Input: part model. Units: mm. Frame: model coordinates. Coordinates: 2 decimals unless noted, no trailing zeros. Write each loop counter-clockwise with the first axis right and the second up, starting at its lowest first coordinate (ties: lowest second). Pieces come first, ordered by that corner, then holes. Notation, with made-up numbers: (59.5, 5) - (74.5, 5) arc R24 cw to (74.5, 35) - close; hole circle Ø7 at (16.25, 21). An arc over 180 degrees is marked (long way). Use CSV: the item, a comma, the result in double quotes.
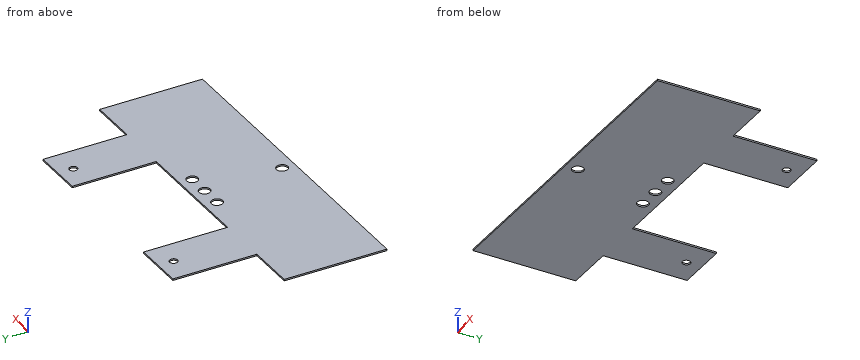
```python
from build123d import *

# Parameters (mm, degrees)
BOSS_EXTRUDE1_DEPTH = 0.6096
SKETCH5_R           = 2.25
CUT_EXTRUDE2_DEPTH  = 430.420105
SKETCH6_R           = 1.5875
CUT_EXTRUDE5_DEPTH  = 0.6096
SKETCH7_R           = 1.5875
CUT_EXTRUDE6_DEPTH  = 0.6096
SKETCH8_R           = 2.25
CUT_EXTRUDE7_DEPTH  = 2.54


with BuildPart() as part:
    # Sketch1 → Boss-Extrude1 (new body)
    with BuildSketch(Plane(origin=(16.997226787, -4.149929847, 204.631375634), x_dir=(0.99656941, 0.00195951, -0.082737969), z_dir=(-0.082760694, 0.020206301, -0.996364578))):
        Polygon((-405.631572024, 283.216979703), (-385.692572024, 283.216979703), (-385.692572024, 323.856979703), (-405.014358213, 323.856979703), (-432.414358217, 323.856979703), (-445.097076418, 323.856979703), (-465.359895626, 323.856979703), (-479.498480719, 323.856979703), (-500.373572024, 323.856979703), (-520.312572024, 323.856979703), (-520.312572024, 283.216979703), (-500.373572024, 283.216979703), (-500.373572024, 250.003685703), (-479.037572024, 250.003685703), (-479.037572024, 283.216979703), (-426.967572024, 283.216979703), (-426.967572024, 250.003685703), (-405.631572024, 250.003685703), align=None)
    extrude(amount=BOSS_EXTRUDE1_DEPTH)

    # Sketch5 → Cut-Extrude2 (cut)
    with BuildSketch(Plane(origin=(16.946775868, -4.137612086, 204.023991787), x_dir=(-0.996569449, -0.001678044, 0.082743681), z_dir=(-0.082760694, 0.020206301, -0.996364578))):
        with Locations((452.956635294, -318.984510283)):
            Circle(SKETCH5_R)
    cut_extrude2 = extrude(amount=-CUT_EXTRUDE2_DEPTH, mode=Mode.SUBTRACT)

    # Mirror1: Cut-Extrude2 across plane
    add(cut_extrude2.mirror(Plane(origin=(0.085159645, -303.474424262, -6.16154314), x_dir=(5.696e-06, -0.020299151, 0.999793951), z_dir=(0.000280558, -0.999793912, -0.020299152))), mode=Mode.SUBTRACT)

    # Sketch6 → Cut-Extrude5 (cut)
    with BuildSketch(Plane(origin=(16.946775868, -4.137612086, 204.023991787), x_dir=(-0.996569449, -0.001678044, 0.082743681), z_dir=(-0.082760694, 0.020206301, -0.996364578))):
        with Locations((416.50680125, -256.173836565)):
            Circle(SKETCH6_R)
    extrude(amount=-CUT_EXTRUDE5_DEPTH, mode=Mode.SUBTRACT)

    # Sketch7 → Cut-Extrude6 (cut)
    with BuildSketch(Plane(origin=(16.946775868, -4.137612086, 204.023991787), x_dir=(-0.996569449, -0.001678044, 0.082743681), z_dir=(-0.082760694, 0.020206301, -0.996364578))):
        with Locations((489.681466673, -256.194436956)):
            Circle(SKETCH7_R)
    extrude(amount=-CUT_EXTRUDE6_DEPTH, mode=Mode.SUBTRACT)

    # Sketch8 → Cut-Extrude7 (cut)
    with BuildSketch(Plane(origin=(16.997226787, -4.149929847, 204.631375634), x_dir=(0.996569449, 0.001678044, -0.082743681), z_dir=(0.082760694, -0.020206301, 0.996364578))):
        with Locations((-443.925718519, -288.341966658)):
            Circle(SKETCH8_R)
        with Locations((-960.270444462, 120.825542597)):
            Circle(SKETCH8_R)
        with Locations((-462.00480383, -288.347056346)):
            Circle(SKETCH8_R)
    extrude(amount=-CUT_EXTRUDE7_DEPTH, mode=Mode.SUBTRACT)


solid = part.part
```
(1) Cut plane B-B on x = -476. Return loops of the section in (y, z).
Check values:
outline,"(-328.91, 238.99) - (-328.9, 238.38) - (-255.06, 239.88) - (-255.07, 240.49) - close"
(2) Cut plane C-C on y = -312. Return loops of the section in (x, z), and give its area (3 significant figures).
Check values:
outline,"(-501.49, 240.84) - (-367.34, 229.7) - (-367.29, 230.31) - (-501.44, 241.45) - close"
area,"82.1 mm^2"
(3) Pin query (flat end, axial travel): pin 1 Ø1 at (x, z) = (-437.5, 236) entering from +Y; pin 2 Ø6 at (y, z) = (-264.5, 238.5) entering from +X; pin 3 Ø2 at (y, z) = (-271, 237) entering from +X; pin 4 Ø1.5 at (x, y) = (-455.5, -297) entering from -Z. Return the tip coordinate at first contact, or that it passes through.
Check values:
pin 1,"y = -288.19"
pin 2,"x = -460.32"
pin 3,"through"
pin 4,"z = 237.26"
(4) Ray query, probe 1 along Z at (x, y) = (-398, -297.5); probe 2 along Z at (x, y) = (-476, -263). Return the intervals inside material, ascending. Write a range as from..to.
Check values:
probe 1,"232.54..233.15"
probe 2,"239.72..240.33"
(5) Cut plane A-A on y = -272.5. Return loops of the section in (x, z).
Check values:
outline,"(-481.64, 240) - (-460.37, 238.23) - (-460.32, 238.84) - (-481.58, 240.6) - close; (-408.48, 233.92) - (-387.22, 232.15) - (-387.17, 232.76) - (-408.43, 234.53) - close"
